Part model, mm, in its own coordinate system. Give positions to 0.01 mm unless a question says otherwise; leave off trailing zeros. Order: outer loops, then holes, each group sorted by start corner. A loop starts at its lowest first (then second) coordinate and runs counter-clockwise, first axis right, second up. Notation, with made-up numbers: M 60.25,12.25 L 103.25,12.25 A19 cw 103.25,26.25 Z; hole C -38,42 d6. An arc over 180 degrees is marked long. Return JSON: item names as keys, results as strings.
Autodesk Inventor part; units mm, degrees
ref_plane "YZ Plane" through (0, 0, 0) normal (1, 0, 0) x (0, 1, 0)
ref_plane "XZ Plane" through (0, 0, 0) normal (0, 1, 0) x (-1, 0, 0)
ref_plane "XY Plane" through (0, 0, 0) normal (0, 0, 1) x (1, 0, 0)
sketch "Sketch1" plane through (0, 0, 0) normal (1, 0, 0) x (0, 1, 0)
  circle A0 centre (0, 0) radius 30
  dimension "d228" = 60
extrude "Extrusion1" add sketch "Sketch1" along normal blind 4
sketch "Sketch3" plane through (4, 0, 0) normal (1, 0, 0) x (0, 0, -1)
  circle A0 centre (0, 0) radius 30
  line L0 (-2.5, 25) -> (2.5, 25)
  line L1 (0, -42) -> (0, 42)
  circle A1 centre (0, 0) radius 7.5
  line L2 (2.5, 25) -> (2.5, 7.0711)
  line L3 (-2.5, 7.0711) -> (-2.5, 25)
  circle A2 centre (0, 0) radius 25
  line L4 (-17.9871, 17.5418) -> (-3.9697, 6.3633)
  line L5 (-21.1045, 13.6327) -> (-17.9871, 17.5418)
  line L6 (-7.0871, 2.4542) -> (-21.1045, 13.6327)
  line L7 (-24.9295, -3.1257) -> (-7.4501, 0.8639)
  line L8 (-23.8169, -8.0003) -> (-24.9295, -3.1257)
  line L9 (-6.3375, -4.0108) -> (-23.8169, -8.0003)
  line L10 (-13.0995, -21.4395) -> (-5.3204, -5.2861)
  line L11 (-8.5947, -23.6089) -> (-13.0995, -21.4395)
  line L12 (-0.8156, -7.4555) -> (-8.5947, -23.6089)
  line L13 (8.5947, -23.6089) -> (0.8156, -7.4555)
  line L14 (13.0995, -21.4395) -> (8.5947, -23.6089)
  line L15 (5.3204, -5.2861) -> (13.0995, -21.4395)
  line L16 (23.8169, -8.0003) -> (6.3375, -4.0108)
  line L17 (24.9295, -3.1257) -> (23.8169, -8.0003)
  line L18 (7.4501, 0.8639) -> (24.9295, -3.1257)
  line L19 (21.1045, 13.6327) -> (7.0871, 2.4542)
  line L20 (17.9871, 17.5418) -> (21.1045, 13.6327)
  line L21 (3.9697, 6.3633) -> (17.9871, 17.5418)
  point P0 (23.6947, -7.9725)
  point P1 (13.0451, -21.3266)
  point P2 (-8.5403, -23.496)
  point P3 (8.5403, -23.496)
  point P4 (0.8156, -7.4555)
  point P5 (-13.0451, -21.3266)
  point P6 (-23.6947, -7.9725)
  point P7 (-24.8073, -3.0978)
  point P8 (-7.4501, 0.8639)
  point P9 (-21.0065, 13.5545)
  point P10 (-17.8891, 17.4637)
  point P11 (-2.5, 24.8747)
  point P12 (17.8891, 17.4637)
  point P13 (2.5, 24.8747)
  point P14 (21.0065, 13.5545)
  point P15 (7.0871, 2.4542)
  point P16 (24.8073, -3.0978)
  dimension "d251" = 15
  dimension "d252" = 5
  dimension "d259" = 5
  dimension "d262" = 360
extrude "Extrusion2" cut sketch "Sketch3" against normal blind 4 contours A2 L12 A1 L1 | L1 A1 L13 A2 | A2 L21 A1 L2 | L3 A1 L4 A2 | L10 A2 L9 A1 | A1 L16 A2 L15 | L19 A2 L18 A1 | A1 L7 A2 L6
properties part number "Langbektang houder"
Q1. Band-saw the part on A-A (y = 10). Give the cut face in (x, z), then the cut area to 3 significant figures.
Established:
{"outline": "M 0,-28.28 L 4,-28.28 L 4,-22.91 L 0,-22.91 Z; M 0,-16.55 L 4,-16.55 L 4,-8.53 L 0,-8.53 Z; M 0,-2.5 L 4,-2.5 L 4,2.5 L 0,2.5 Z; M 0,8.53 L 4,8.53 L 4,16.55 L 0,16.55 Z; M 0,22.91 L 4,22.91 L 4,28.28 L 0,28.28 Z", "area": "127 mm²"}
Q2. Pin check, flat tips, straight feed: pin 1 (1.5 mm diameter, centred on x = 0.5, z = 21, fed in from -Y); pin 2 (2 mm diameter, centred on x = 3, z = 7, fed in from +Y); pin 3 (4 mm diameter, centred on y = -23, z = -22.5, fed in from +X) (3 decimals); pin 4 (2 mm diameter, centred on x = 2.5, y = 13, fed in from -Z). Stop position of each tip, or through.
Established:
{"pin 1": "stops at y = -22.13", "pin 2": "stops at y = 29.39", "pin 3": "passes through", "pin 4": "stops at z = -27.5"}
Q3. Band-saw the part on B-B (x = 1.75). Give the number of separate pieces and of enclosed holes in the cut face, then the cut area to 3 significant figures.
Established:
{"separate pieces": "1", "enclosed holes": "7", "area": "1,660 mm²"}
Q4. Band-saw the part on C-C (y = 4). Give the cut face in (x, z).
Established:
{"outline": "M 0,-29.73 L 4,-29.73 L 4,-24.68 L 0,-24.68 Z; M 0,-9.03 L 4,-9.03 L 4,9.03 L 0,9.03 Z; M 0,24.68 L 4,24.68 L 4,29.73 L 0,29.73 Z"}
Q5. Two-plate mould, pull along Z, no slides. Class faces 1 (the flat face through (2, 16, 2.5)), 2 (the cylindrical face through (1.97, -29.97, -1.32)), 3 (the flat face through (4, 0, 0)): +Z half, -Z half, draft (parallel to the pull), parting line (faces both ways), or undercut.
Established:
{"face 1": "undercut", "face 2": "parting line", "face 3": "draft"}
Q6. Probe line 1 along Z through (x, y) = (2.4, 3); line 2 along Y through (x, z) = (3.85, -8); line 3 along Z through (x, y) = (3.05, 19.5). List the from-to ranges inside material, lowest first.
Established:
{"line 1": "z = -29.85 to -24.82, -7.77 to 7.77, 24.82 to 29.85", "line 2": "y = -28.91 to -23.69, -22.37 to -10.85, -4.39 to 0.74, 3.18 to 9.58, 23.69 to 28.91", "line 3": "z = -22.8 to -15.64, -2.5 to 2.5, 15.64 to 22.8"}
Q7. Band-saw the part on D-D (y = -9.5). Give the cut face in (x, z).
Established:
{"outline": "M 0,-28.46 L 4,-28.46 L 4,-23.12 L 0,-23.12 Z; M 0,-7.35 L 4,-7.35 L 4,-1.8 L 0,-1.8 Z; M 0,1.8 L 4,1.8 L 4,7.35 L 0,7.35 Z; M 0,23.12 L 4,23.12 L 4,28.46 L 0,28.46 Z"}
